Autodesk Inventor part; units mm, degrees
ref_plane "Work Plane1" through (0, 0, 6.5) normal (0, 0, 1) x (1, 0, 0)
ref_plane "Work Plane2" through (0, 0, 6.5) normal (0, 0, -1) x (-1, 0, 0)
ref_plane "YZ Plane" through (0, 0, 0) normal (1, 0, 0) x (0, 1, 0)
sketch "Sketch1" plane through (0, 0, 0) normal (0, 0, 1) x (1, 0, 0)
  line L0 (-5, 5) -> (5, 5)
  line L1 (5, 5) -> (5, -5)
  line L2 (5, -5) -> (-5, -5)
  line L3 (-5, -5) -> (-5, 5)
  line L4 (-5, 5) -> (5, -5) construction
  line L5 (5, 5) -> (-5, -5) construction
  point P0 (0, 0)
  dimension "d0" = 10
  dimension "d1" = 10
extrude "Extrusion1" add sketch "Sketch1" along normal blind 13
sketch "Sketch2" plane through (0, 0, 13) normal (0, 0, 1) x (1, 0, 0)
  circle A0 centre (0, 0) radius 2.35
  dimension "d4" = 4.7
extrude "Extrusion2" add sketch "Sketch2" along normal blind 10
ref_plane "Work Plane1" through (0, 0, 6.5) normal (0, 0, 1) x (1, 0, 0)
mirror "Mirror1" about plane through (0, 0, 6.5) normal (0, 0, 1) of "Extrusion2"
sketch "Sketch3" plane through (-5, 5, 0) normal (0, 1, 0) x (1, 0, 0)
  line L0 (0, 0) -> (0, -13)
  line L1 (0, -6.5) -> (10, -6.5)
  line L2 (10, 0) -> (10, -13)
  circle A0 centre (5, -6.5) radius 3
  point P0 (5, 0)
  dimension "d7" = 6
extrude "Extrusion3" cut sketch "Sketch3" against normal through all
sketch "Sketch4" plane through (5, -5, 0) normal (1, 0, 0) x (0, 0, -1)
  line L0 (0, 0) -> (0, 10)
  line L1 (0, 10) -> (-13, 10)
  line L2 (-13, 0) -> (-13, 10)
  line L3 (0, 0) -> (-13, 0)
  point P0 (0, 5)
extrude "Extrusion4" add sketch "Sketch4" along normal blind 70
mirror "Mirror2" about plane through (0, 0, 0) normal (1, 0, 0) of "Extrusion4"
sketch "Sketch5" plane through (0, 0, 13) normal (0, 0, 1) x (1, 0, 0)
  line L0 (-75, 5) -> (75, 5)
  line L1 (0, 5) -> (0, -5)
  line L2 (75, -5) -> (-75, -5)
  line L3 (-75, 5) -> (-75, -5)
  line L4 (-75, -5) -> (-75, 5)
  line L5 (-60, -5) -> (-60, 5)
  line L6 (75, 5) -> (75, -5)
  line L7 (60, -5) -> (60, 5)
  point P0 (0, 0)
  dimension "d12" = 15
extrude "Extrusion5" add sketch "Sketch5" along normal blind 15 contours L0 L5 L2 L3 | L0 L6 L2 L7
ref_plane "Work Plane2" through (0, 0, 6.5) normal (0, 0, -1) x (-1, 0, 0)
mirror "Mirror3" about plane through (0, 0, 6.5) normal (0, 0, -1) of "Extrusion5"
sketch "Sketch6" plane through (-75, -5, 28) normal (-1, 0, 0) x (0, 0, 1)
  line L0 (-28, 10) -> (-43, 10)
  line L1 (-15, 10) -> (0, 10)
  line L2 (0, 10) -> (-43, 10)
  line L3 (-28, 10) -> (-43, 10)
  line L4 (-35.5, 10) -> (-35.5, 15)
  circle A0 centre (-35.5, 15) radius 2.5
  circle A1 centre (-35.5, 15) radius 5
  line L5 (-40.5, 15) -> (-40.5, 10)
  line L6 (-30.5, 15) -> (-30.5, 10)
  line L7 (-40.5, 10) -> (-30.5, 10)
  line L8 (-18.5, 0) -> (-24.5, 0)
  line L9 (-21.5, 0) -> (-21.5, 20.3601)
  line L10 (-15, 10) -> (0, 10)
  line L11 (-7.5, 10) -> (-7.5, 15)
  circle A2 centre (-7.5, 15) radius 2.5
  circle A3 centre (-7.5, 15) radius 5
  line L12 (-2.5, 15) -> (-2.5, 10)
  line L13 (-12.5, 15) -> (-12.5, 10)
  point P0 (-28, 5)
  dimension "d15" = 5
  dimension "d16" = 5
  dimension "d17" = 10
extrude "Extrusion6" add sketch "Sketch6" against normal blind 6
mirror "Mirror4" about plane through (0, 0, 0) normal (1, 0, 0) of "Extrusion6"
sketch "Sketch8" plane through (0, 0, 0) normal (0, 0, -1) x (-1, 0, 0)
  line L0 (3, -96.3437) -> (3, 27.6563)
  line L1 (60, 5) -> (-60, 5)
  line L2 (3, 5) -> (8, 5)
  line L3 (8, 5) -> (8, 10)
  circle A0 centre (13, 10) radius 5
  line L4 (60, 5) -> (-60, 5)
  line L5 (18, 10) -> (18, 5)
  circle A1 centre (13, 10) radius 2.5
  point P0 (0, 0)
  dimension "d22" = 10
  dimension "d20" = 5
  dimension "d21" = 5
  dimension "d23" = 5
extrude "Extrusion7" add sketch "Sketch8" against normal blind 6
sketch "Sketch9" plane through (0, 0, 6) normal (0, 0, 1) x (1, 0, 0)
  arc A0 (-8, 10) -> (-18, 10) centre (-13, 10) ccw
  line L0 (-18, 10) -> (-8, 10)
  point P0 (0, 0)
extrude "Extrusion8" add sketch "Sketch9" against normal up to surface (6 mm away)
properties part number "Claw Connector 2"
Part model, mm, in its own coordinate system. A direction names the side the tool comes from. Coordinates: 2 decimals unless noted, no trailing zeros. Write each loop counter-clockwise with the first axis right and the second up, starting at its lowest first coordinate (ties: lowest second). Pieces come first, ordered by that corner, then holes. Notation, with made-up numbers: (-29.5, -16) - (22.5, -16) arc R25 ccw to (22.5, 20) - close; hole circle Ø10 at (0.25, -19.75). An arc over 180 degrees is marked (long way). Put each result on its own line as item: value.
1. Flat gauge pins, fed straight in: pin 1 Ø6 at (y, z) = (10, 20.5) entering from -X; pin 2 Ø4 at (x, y) = (-70.5, 8) entering from +Z; pin 3 Ø3 at (x, y) = (-7, 2) entering from +Z; pin 4 Ø12 at (x, y) = (-19, 12) entering from +Z. Where does each tip first touch, or does it go through?
Final values:
pin 1: stops at x = -75
pin 2: stops at z = 25.5
pin 3: stops at z = 13
pin 4: stops at z = 6
2. Two-plate mould, pull along Z, no slides. Class faces 5 (the flat face through (-69, 9, -10)), 6 (the flat face through (72, 7, -2.5)), 7 (the flat face through (67, 0, 28)): +Z half, -Z half, draft (parallel to the pull), parting line (faces both ways), or undercut.
Final values:
face 5: draft
face 6: undercut
face 7: +Z half
3. Band-saw the part on B-B (x = -13). Write the cut outline in (y, z).
Final values:
outline: (-5, 0) - (7.5, 0) - (7.5, 6) - (5, 6) - (5, 13) - (-5, 13) - close; (10, 0) - (15, 0) - (15, 6) - (10, 6) - close
4. 3-axis set-ups, long thin cutter, end or side, ignore diameter. For faces 1 (the flat face through (69, 9, -5)), 2 (the flat face through (-72, 8, -12.5)), 3 (the flat face through (60, 0, -7)), 4 (the flat face through (-72, 8, -2.5)): which of +Z, -Z, +X, -X, +Y, -Y reach the whole face in a straight line?
Final values:
face 1: +Z, -Z, +Y
face 2: -Z, +X, -X, +Y
face 3: -Z, +Y, -Y
face 4: +X, -X, +Y
5. Probe line 1 along Z through (x, y) = (71, 10); line 2 along Z through (x, y) = (0, -1.75); line 3 along X through (y, z) = (-2.5, 15). List the from-to ranges inside material, lowest first. Write a range as [from, to].
Final values:
line 1: z = [-12.5, -10], [-5, -2.5], [15.5, 18], [23, 25.5]
line 2: z = [-10, 3.5], [9.5, 23]
line 3: x = [-75, -60], [60, 75]
6. Band-saw the part on A-A (z = 20.5). Write the cut outline in (x, y).
Final values:
outline: (-75, -5) - (-60, -5) - (-60, 5) - (-69, 5) - (-69, 7.5) - (-75, 7.5) - close; (-75, 12.5) - (-69, 12.5) - (-69, 15) - (-75, 15) - close; circle Ø4.7 at (0, 0); (60, -5) - (75, -5) - (75, 7.5) - (69, 7.5) - (69, 5) - (60, 5) - close; (69, 12.5) - (75, 12.5) - (75, 15) - (69, 15) - close
7. Band-saw the part on D-D (x = -49). Write the cut outline in (y, z), then the cut area to 3 significant figures.
Final values:
outline: (-5, 0) - (5, 0) - (5, 13) - (-5, 13) - close
area: 130 mm²
8. Band-saw the part on C-C (y = 0). Write the cut outline in (x, z), then the cut area to 3 significant figures.
Final values:
outline: (-75, -15) - (-60, -15) - (-60, 0) - (-2.35, 0) - (-2.35, -10) - (2.35, -10) - (2.35, 0) - (60, 0) - (60, -15) - (75, -15) - (75, 28) - (60, 28) - (60, 13) - (2.35, 13) - (2.35, 23) - (-2.35, 23) - (-2.35, 13) - (-60, 13) - (-60, 28) - (-75, 28) - close; hole circle Ø6 at (0, 6.5)
area: 2,920 mm²
